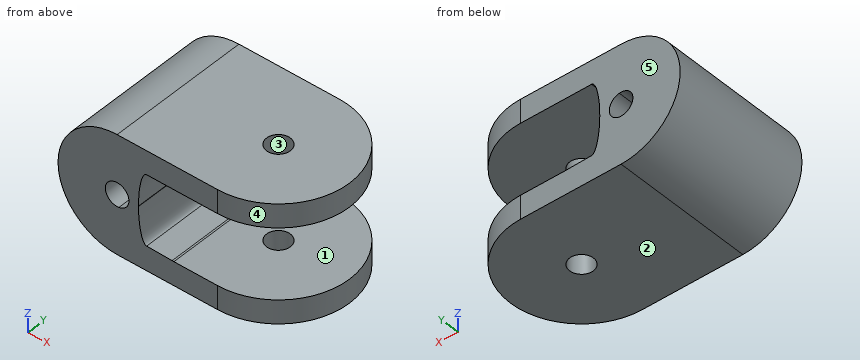
from build123d import *

# Parameters (mm, degrees)
SKETCH1_R               = 125
SKETCH1_R_2             = 25
BOSS_EXTRUDE1_DEPTH     = 300
SKETCH2_R               = 25
BOSS_EXTRUDE2_DEPTH     = 125
CUT_EXTRUDE2_DEPTH      = 75
BOSS_EXTRUDE3_DEPTH     = 300
SKETCH6_R               = 25
CUT_EXTRUDE3_DEPTH      = 487.858552354
CUT_EXTRUDE4_DEPTH      = 487.858552354
CUT_EXTRUDE4_DEPTH_BACK = 487.858552354


with BuildPart() as part:
    # Sketch1 → Boss-Extrude1 (new body)
    with BuildSketch(Plane(origin=(0, 0, 0), x_dir=(1, 0, 0), z_dir=(0, 1, 0))):
        with Locations(Location((0, 0, 0), (0, 0, 270))):
            Circle(SKETCH1_R)
        with Locations(Location((0, 0, 0), (0, 0, 270))):
            Circle(SKETCH1_R_2, mode=Mode.SUBTRACT)
    extrude(amount=BOSS_EXTRUDE1_DEPTH)

    # Sketch2 → Boss-Extrude2 (add, symmetric)
    with BuildSketch(Plane.XY):
        with BuildLine():
            Line((0, 300), (0, 0))
            Line((0, 0), (212.5, 0))
            ThreePointArc((212.5, 0), (362.5, 150), (212.5, 300))
            Line((212.5, 300), (0, 300))
        make_face()
        with Locations((212.5, 150)):
            Circle(SKETCH2_R, mode=Mode.SUBTRACT)
    extrude(amount=BOSS_EXTRUDE2_DEPTH, both=True)

    # Sketch4 → Cut-Extrude2 (cut, symmetric)
    with BuildSketch(Plane.XY):
        with BuildLine():
            Line((3.772306617, 300), (3.772306617, 0))
            Line((3.772306617, 0), (150, 0))
            ThreePointArc((150, 0), (375, 150), (150, 300))
            Line((150, 300), (3.772306617, 300))
        make_face()
    extrude(amount=CUT_EXTRUDE2_DEPTH, both=True, mode=Mode.SUBTRACT)

    # Sketch5 → Boss-Extrude3 (add, through all)
    with BuildSketch(Plane(origin=(0, 0, 0), x_dir=(1, 0, 0), z_dir=(0, 1, 0))):
        with BuildLine():
            Line((120, 75), (3.772306617, 75))
            Line((3.772306617, 75), (3.772306617, 24.713755336))
            ThreePointArc((3.772306617, 24.713755336), (18.964541458, 16.28944957), (25, 0))
            ThreePointArc((25, 0), (18.964541458, -16.28944957), (3.772306617, -24.713755336))
            Line((3.772306617, -24.713755336), (3.772306617, -75))
            Line((3.772306617, -75), (120, -75))
            ThreePointArc((120, -75), (45, 0), (120, 75))
        make_face()
    extrude(amount=BOSS_EXTRUDE3_DEPTH)

    # Sketch6 → Cut-Extrude3 (cut, through all)
    with BuildSketch(Plane(origin=(0, 300, 0), x_dir=(1, 0, 0), z_dir=(0, 1, 0))):
        with Locations(Location((0, 0, 0), (0, 0, 270))):
            Circle(SKETCH6_R)
    extrude(amount=-CUT_EXTRUDE3_DEPTH, mode=Mode.SUBTRACT)

    # Sketch10 → Cut-Extrude4 (cut, two sides: drawn at the far end of the back side and taken through both)
    with BuildSketch(Plane(origin=(0, 0, 0), x_dir=(1, 0, 0), z_dir=(0, 1, 0)).offset(-CUT_EXTRUDE4_DEPTH_BACK)):
        with BuildLine():
            Line((62.5, 73.562310608), (120, 75))
            Line((120, 75), (120, -75))
            Line((120, -75), (62.5, -75))
            add(Edge.make_bspline(
                [(62.5, 73.562310608), (45, 73.562310608), (45, -0.718844696), (45, -75), (62.5, -75)],
                knots=[0, 0, 0, 1.570796327, 1.570796327, 3.141592654, 3.141592654, 3.141592654], degree=2, weights=[1, 0.707106781, 1, 0.707106781, 1]))
        make_face()
    extrude(amount=CUT_EXTRUDE4_DEPTH + CUT_EXTRUDE4_DEPTH_BACK, mode=Mode.SUBTRACT)


solid = part.part
Work out the finished part from the listing and answer in its coordinate system (mm). Face numbers are marked on the shaded views. A direction names the side the tool comes from. Round coordinates to 2 decimals unless told otherwise and drop trailing zeros. Order: outer loops, then holes, each group sorted by start corner. A loop starts at its lowest first (then second) coordinate and runs counter-clockwise, first axis right, second up. Notation, with made-up numbers: M 40,23 L 76,23 A21 ccw 76,58 Z; hole C 61.25,7 d4. An arc over 180 degrees is marked long. Put each result on its own line as item: value. Start each with the question number.
Q1. Straight lines are drawn through the part: L1, parallel to Y at x = 212.5, z = -103.5; L2, parallel to Z at x = 0, y = 144; L3, parallel to Z at x = 199, y = 60.5. For each, find the intervals that lie inside material, in ascending order. Write a range as [from, to].
Q2. Section A-A, the plane x = 178.5 is taken. Write down the section's boundary in (y, z), and give its area (3 significant figures).
Q3. Section C-C, the plane y = 167 is taken. Give the number of separate pieces and of enclosed holes in the cut face, and give its area (3 significant figures).
Q4. Section D-D, the plane x = 298 is taken. Write down the section's boundary in (y, z), and give its area (3 significant figures).
Q5. A tool of negligible diameter and unlimited length cuts with its end or side. For the marked faces 1 and 2, from which of +Z, -Z, +X, -X, +Y, -Y can it reach the whole face along a straight path? Write none if from no direction.
Q6. Flat-ended cylindrical pins translate along their axes: pin 1 (8 mm diameter, centred on y = 196.5, z = 31.5, fed in from -X); pin 2 (6 mm diameter, centred on y = 64.5, z = -97, fed in from +X); pin 3 (4 mm diameter, centred on x = -9.5, y = 211.5, fed in from +Z). Find the tip coordinate at first contact, or state that the pin passes through.
Q7. For a pull along Y with two mould halves and no side action, classify the marked faces 3, 4 and 5 as pulls with the +Y half, pulls with the -Y half, needs draft (parallel to the pull), parting line crosses it, or undercut.
Q8. Section B-B, the plane z = 89 is taken. Write down the section's boundary in (x, y).
Findings below:
1. L1: y = [0, 125], [175, 300]
1. L2: z = [-125, -25], [25, 125]
1. L3: z = [-125, -75], [75, 125]
2. outline: M 0,-125 L 300,-125 L 300,-75 L 0,-75 Z; M 0,75 L 300,75 L 300,125 L 0,125 Z
2. area: 30,000 mm^2
3. separate pieces: 3
3. enclosed holes: 1
3. area: 62,400 mm^2
4. outline: M 26.75,-125 L 273.25,-125 L 273.25,-75 L 26.75,-75 Z; M 26.75,75 L 273.25,75 L 273.25,125 L 26.75,125 Z
4. area: 24,600 mm^2
5. face 1: +X, +Y, -Y
5. face 2: -Z, +X, -X, +Y, -Y
6. pin 1: stops at x = -121.94
6. pin 2: stops at x = 337.77
6. pin 3: stops at z = 124.77
7. face 3: undercut
7. face 4: parting line crosses it
7. face 5: pulls with the +Y half
8. outline: M -87.77,0 L 212.5,0 A150 ccw 212.5,300 L -87.77,300 Z; hole C 212.5,150 d50
